from build123d import *

# Parameters (mm, degrees)
SKETCH1_W           = 38.1
SKETCH1_H           = 38.1
BOSS_EXTRUDE1_DEPTH = 8.89
SKETCH3_W           = 38.1
SKETCH3_H           = 12.7
CUT_EXTRUDE1_DEPTH  = 3.81
SKETCH4_R           = 1.27
CUT_EXTRUDE2_DEPTH  = 28.415532094
SKETCH6_W           = 19.05
SKETCH6_H           = 31.75
CUT_EXTRUDE5_DEPTH  = 29.369651038
CUT_EXTRUDE6_DEPTH  = 12.7
SKETCH8_W           = 38.1
SKETCH8_H           = 19.05
CUT_EXTRUDE7_DEPTH  = 5.08
SKETCH9_R           = 3.2639
CUT_EXTRUDE8_DEPTH  = 29.369651038
CUT_EXTRUDE9_REACH  = 29.416
SKETCH10_R          = 1.5
CHAMFER6_SIZE       = 5.08
CHAMFER7_SIZE       = 3.81
CHAMFER8_SIZE       = 2.54
CHAMFER9_SIZE       = 2.54


with BuildPart() as part:
    # Sketch1 → Boss-Extrude1 (new body)
    with BuildSketch(Plane.XY):
        Rectangle(SKETCH1_W, SKETCH1_H)
    extrude(amount=-BOSS_EXTRUDE1_DEPTH)

    # Sketch3 → Cut-Extrude1 (cut)
    with BuildSketch(Plane.XY):
        with Locations((0, 12.7)):
            Rectangle(SKETCH3_W, SKETCH3_H)
    extrude(amount=-CUT_EXTRUDE1_DEPTH, mode=Mode.SUBTRACT)

    # Sketch4 → Cut-Extrude2 (cut, through all)
    with BuildSketch(Plane.XY.offset(-3.81)):
        with Locations((-13, 16.002)):
            Circle(SKETCH4_R)
        with Locations(Location((13, 16.002, 0), (0, 0, 180))):
            Circle(SKETCH4_R)
    extrude(amount=-CUT_EXTRUDE2_DEPTH, mode=Mode.SUBTRACT)

    # Sketch6 → Cut-Extrude5 (cut, through all)
    with BuildSketch(Plane.XY):
        with Locations((0, 9.525)):
            Rectangle(SKETCH6_W, SKETCH6_H)
    extrude(amount=-CUT_EXTRUDE5_DEPTH, mode=Mode.SUBTRACT)

    # Sketch7 → Cut-Extrude6 (cut)
    with BuildSketch(Plane(origin=(0, 19.05, 0), x_dir=(1, 0, 0), z_dir=(0, 1, 0))):
        Polygon((15.882742773, 7.323143279), (-15.866364793, 7.561195322), (-15.882742773, 5.376856721), (15.866364793, 5.138804678), align=None)
    extrude(amount=-CUT_EXTRUDE6_DEPTH, mode=Mode.SUBTRACT)

    # Sketch8 → Cut-Extrude7 (cut)
    with BuildSketch(Plane(origin=(0, 0, -8.89), x_dir=(-1, 0, 0), z_dir=(0, 0, -1))):
        with Locations((0, -9.525)):
            Rectangle(SKETCH8_W, SKETCH8_H)
    extrude(amount=-CUT_EXTRUDE7_DEPTH, mode=Mode.SUBTRACT)

    # Sketch9 → Cut-Extrude8 (cut, through all)
    with BuildSketch(Plane.XY):
        with Locations((0, -12.7)):
            Circle(SKETCH9_R)
    extrude(amount=-CUT_EXTRUDE8_DEPTH, mode=Mode.SUBTRACT)

    # Cut-Extrude9: up to this plane
    cut_extrude9_end = Plane(origin=(15.866364793, 6.35, -5.138804678), z_dir=(-0.007497702129822743, 0, 0.9999718918363518))
    # Sketch10 → Cut-Extrude9 (cut, up to the surface)
    with BuildSketch(Plane.XY.offset(-3.81), mode=Mode.PRIVATE) as cut_extrude9_sk1:
        with Locations((-13, 16.002)):
            Circle(SKETCH10_R)
    cut_extrude9_tool1 = split(extrude(cut_extrude9_sk1.sketch, amount=-CUT_EXTRUDE9_REACH, mode=Mode.PRIVATE), bisect_by=cut_extrude9_end, keep=Keep.BOTH, mode=Mode.PRIVATE)
    add(cut_extrude9_tool1.solids().sort_by_distance((-13, 16.002, -3.81))[0], mode=Mode.SUBTRACT)
    # Sketch10 → Cut-Extrude9 (cut, up to the surface)
    with BuildSketch(Plane.XY.offset(-3.81), mode=Mode.PRIVATE) as cut_extrude9_sk2:
        with Locations((13, 16.002)):
            Circle(SKETCH10_R)
    cut_extrude9_tool2 = split(extrude(cut_extrude9_sk2.sketch, amount=-CUT_EXTRUDE9_REACH, mode=Mode.PRIVATE), bisect_by=cut_extrude9_end, keep=Keep.BOTH, mode=Mode.PRIVATE)
    add(cut_extrude9_tool2.solids().sort_by_distance((13, 16.002, -3.81))[0], mode=Mode.SUBTRACT)

    # Chamfer6
    chamfer6_edges = [part.edges().sort_by_distance(p)[0] for p in [
        (-14.2875, 0, -3.81),
        (14.2875, 0, -3.81),
    ]]
    chamfer(chamfer6_edges, length=CHAMFER6_SIZE - 0.0001)  # a hair under: the kernel refuses the full size

    # Chamfer7
    chamfer7_edges = [part.edges().sort_by_distance(p)[0] for p in [
        (-14.2875, 6.35, -3.81),
        (14.2875, 6.35, -3.81),
    ]]
    chamfer(chamfer7_edges, length=CHAMFER7_SIZE - 0.0001)  # a hair under: the kernel refuses the full size

    # Chamfer8
    chamfer8_edges = [part.edges().sort_by_distance(p)[0] for p in [
        (-9.525, 0, 0),
        (0, -6.35, 0),
        (9.525, 0, 0),
    ]]
    chamfer(chamfer8_edges, length=CHAMFER8_SIZE)

    # Chamfer9
    chamfer9_edges = [part.edges().sort_by_distance(p)[0] for p in [
        (-19.05, -19.05, -1.905),
        (19.05, -19.05, -1.905),
        (0, -19.05, -3.81),
    ]]
    chamfer(chamfer9_edges, length=CHAMFER9_SIZE)


solid = part.part
Here's how the part is built. I have some questions about the finished solid (model axes, mm). A direction names the side the tool comes from. Give positions to 0.01 mm unless a question says otherwise; leave off trailing zeros. Loops run counter-clockwise (first coordinate to the right, second up) from the corner with the lowest first, then second, coordinate; pieces in that order, holes last. Notation, with made-up numbers: (9, -3) -> (31, -3) arc R28 ccw to (31, 28) -> close; hole circle Ø5 at (-28.75, 83). An arc over 180 degrees is marked (long way). Answer as a JSON object with one key per item and string values. Group by question number.
Item 1: On a 3-axis mill with a long thin cutter (end or side, diameter ignored), from which of +Z, -Z, +X, -X, +Y, -Y can I reach the whole of each face in a straight line? I mean faces 1 (the flat face through (9.525, 6, -6)), 2 (the flat face through (14.35, -2.5, -6.39)), 3 (the flat face through (-10.777, -0.125, -1.288)). Say none if no direction works.
Item 2: Will these pins go through, and if not, where does the flat tip stop? pin 1 (4 mm diameter, centred on x = 14, z = -7, fed in from -Y); pin 2 (5 mm diameter, centred on x = -13, y = 16.002, fed in from +Z); pin 3 (3.5 mm diameter, centred on x = -13, y = 16.002, fed in from -Z); pin 4 (1 mm diameter, centred on x = 8, z = -4, fed in from -Y).
Item 3: Thinking about a two-plate mould opening in Y: for faces 4 (the flat face through (-0.17, -7.6, -1.29)), 5 (the cylindrical face through (12.67, 14.54, -4.48)), 6 (the flat face through (0, -9, -3.81)), which applies, pulls with the +Y half, pulls with the -Y half, needs draft (parallel to the pull), parting line crosses it, or undercut?
Item 4: Imagine slicing it at A-A on x = 0. Write out the boundary of the cut face in (y, z).
Item 5: Imagine slicing it at B-B on y = 5.5. Write out the boundary of the cut face in (x, z) (3 decimals), then the cut area to 3 significant figures.
Item 6: Imagine slicing it at C-C on z = -3. Write out the boundary of the cut face in (x, y) (3 decimals), then the cut area to 3 significant figures.
Item 7: I need wall thicknesses on L1, parallel to X at y = -12.5, z = -3.25; L2, parallel to X at y = 1, z = -3.5 (3 decimals); L3, parallel to Z at x = -11, y = -12. Which ranges of each line are inside material? Lowest first, please.
Item 8: Imagine slicing it at D-D on x = 13. Give the number of separate pieces and of enclosed holes in the cut face, then the cut area to 3 significant figures.
Answer list:
{
 "1": {"face 1": "+Z, -Z, +Y", "face 2": "-Z, +X, -X, -Y", "face 3": "+Z, +Y"},
 "2": {"pin 1": "stops at y = -3.89", "pin 2": "stops at z = -3.81", "pin 3": "stops at z = -8.89", "pin 4": "stops at y = -16.82"},
 "3": {"face 4": "pulls with the +Y half", "face 5": "undercut", "face 6": "needs draft"},
 "4": {"outline": "(-19.05, -1.27) -> (-16.51, -3.81) -> (-15.96, -3.81) -> (-15.96, 0) -> (-19.05, 0) -> close; (-9.44, -3.81) -> (-6.35, -3.81) -> (-6.35, -2.54) -> (-8.89, 0) -> (-9.44, 0) -> close"},
 "5": {"outline": "(-19.05, -8.89) -> (-9.525, -8.89) -> (-9.525, -2.54) -> (-12.065, 0) -> (-19.05, 0) -> close; (9.525, -8.89) -> (19.05, -8.89) -> (19.05, 0) -> (12.065, 0) -> (9.525, -2.54) -> close", "area": "163 mm2"},
 "6": {"outline": "(-19.05, -16.51) -> (-18.24, -17.32) -> (18.24, -17.32) -> (19.05, -16.51) -> (19.05, 9.35) -> (9.525, 9.35) -> (9.525, -6.35) -> (-9.525, -6.35) -> (-9.525, 9.35) -> (-19.05, 9.35) -> close; hole circle Ø6.528 at (0, -12.7)", "area": "683 mm2"},
 "7": {"L1": "x = -19.05 to -3.26, 3.26 to 19.05", "L2": "x = -19.05 to -9.525, 9.525 to 19.05", "L3": "z = -3.81 to 0"},
 "8": {"separate pieces": "3", "enclosed holes": "0", "area": "175 mm2"}
}
